from build123d import *

# Parameters (mm, degrees)
BOSS_EXTRUDE1_DEPTH = 6
SKETCH2_R           = 2.5
SKETCH2_W           = 20
SKETCH2_H           = 20
CUT_EXTRUDE3_DEPTH  = 6


with BuildPart() as part:
    # Sketch1 → Boss-Extrude1 (new body)
    with BuildSketch(Plane(origin=(0, 0, 0), x_dir=(1, 0, 0), z_dir=(0, 1, 0))):
        Polygon((-25, 11), (25, 11), (25, -11), (25, -40), (20.004090827, -40), (20.004090827, -46), (11.004090827, -46), (11.004090827, -40), (2.05, -40), (2.05, -38), (4, -38), (4, -33), (2.05, -33), (2.05, -27), (-2.05, -27), (-2.05, -33), (-4, -33), (-4, -38), (-2.05, -38), (-2.05, -40), (-11.004090827, -40), (-11.004090827, -46), (-20.004090827, -46), (-20.004090827, -40), (-25, -40), (-25, -11), align=None)
    extrude(amount=BOSS_EXTRUDE1_DEPTH)

    # Sketch2 → Cut-Extrude3 (cut)
    with BuildSketch(Plane(origin=(0, 0, 0), x_dir=(1, 0, 0), z_dir=(0, 1, 0))):
        with Locations((-20, 0)):
            Circle(SKETCH2_R)
        with Locations((20, 0)):
            Circle(SKETCH2_R)
        Rectangle(SKETCH2_W, SKETCH2_H)
    extrude(amount=CUT_EXTRUDE3_DEPTH, mode=Mode.SUBTRACT)


solid = part.part
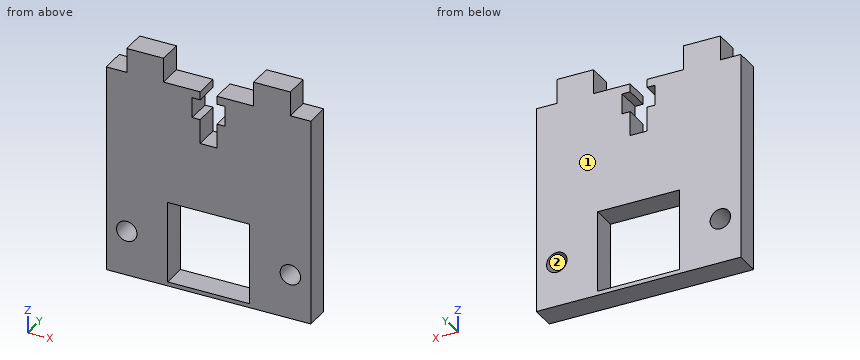
Verification items for the finished model (mm, model axes). Face numbers are marked on the shaded views. Give positions to 0.01 mm unless a question says otherwise; leave off trailing zeros. Write each loop counter-clockwise with the first axis right and the second up, starting at its lowest first coordinate (ties: lowest second). Pieces come first, ordered by that corner, then holes.
(1) Cross-section at A-A (z = 0). Enter the section's corners in (x, y).
(2) Cross-section at C-C (y = 2.1). State how many separate pieces and enclosed holes the cut face has, plus the area to 3 significant figures.
(3) Mould release check, pull along X, two halves, no side actions. Record for the marked faces 1 and 2: +X half, -X half, draft (parallel to the pull), parting line (faces both ways), or undercut.
(4) Gauge pin test, flat ends, axial feed: pin 1 (3 mm diameter, centred on x = -1, y = 4, fed in from +Z); pin 2 (3 mm diameter, centred on y = 1.5, z = 43, fed in from -X). Record the tip position at first contact, or that the pin passes through.
(5) Material ranges on line 1 (X direction, y = 3.1, z = 0); line 2 (X direction, y = 5.75, z = 41.5); line 3 (X direction, y = 3.75, z = 28), recorded low to high.
(6) Cross-section at B-B (x = -5). Enter the section's corners in (y, z).
Worked out:
1. outline: (-25, 0) - (-22.5, 0) - (-22.5, 6) - (-25, 6) - close; (-17.5, 0) - (-10, 0) - (-10, 6) - (-17.5, 6) - close; (10, 0) - (17.5, 0) - (17.5, 6) - (10, 6) - close; (22.5, 0) - (25, 0) - (25, 6) - (22.5, 6) - close
2. separate pieces: 1
2. enclosed holes: 3
2. area: 2,150 mm2
3. face 1: draft
3. face 2: undercut
4. pin 1: stops at z = 40
4. pin 2: stops at x = -20
5. line 1: x = -25 to -22.5, -17.5 to -10, 10 to 17.5, 22.5 to 25
5. line 2: x = -20 to -11, 11 to 20
5. line 3: x = -25 to -2.05, 2.05 to 25
6. outline: (0, -11) - (6, -11) - (6, -10) - (0, -10) - close; (0, 10) - (6, 10) - (6, 40) - (0, 40) - close
